Can you work these out from the model? Positions are in its coordinate system, mm. A direction names the side the tool comes from. Coordinates: 2 decimals unless noted, no trailing zeros. Loops run counter-clockwise (first coordinate to the right, second up) from the corner with the lowest first, then second, coordinate; pieces in that order, holes last. Notation, with made-up numbers: M 72.25,-2 L 121.25,-2 A22 cw 121.25,11 Z; hole C 7.5,40 d10. An arc over 180 degrees is marked long. Answer as a JSON object with one key per item and string values. Group by question number.
Item 1: Suppose I cut it at B-B (z = 17.25). Write out the boundary of the cut face in (x, y), then the cut area to 3 significant figures.
Item 2: We'd pull the mould along X, two halves only. Please class faces 4 (the flat face through (-6, 18.562, 15)), 5 (the flat face through (11, -7, 2)), 6 (the cylindrical face through (63.75, 1.4, 4.44)): +X half, -X half, draft (parallel to the pull), parting line (faces both ways), or undercut.
Item 3: Suppose I cut it at C-C (x = -7.5). Write out the boundary of the cut face in (y, z).
Item 4: I'm going to push flat-ended pins straight in: pin 1 Ø8 at (y, z) = (-8, 4.5) entering from -X; pin 2 Ø6.5 at (x, y) = (25, 0) entering from -Z; pin 3 Ø1.2 at (y, z) = (10, 3.5) entering from -X; pin 4 Ø3 at (x, z) = (19, 3.5) entering from -Y. Where does each tip first touch, or does it pass through?
Item 5: If I drill on line 1 (X direction, y = -3.5, z = 14.25); line 2 (Y direction, x = 62.25, z = 13.5); line 3 (Y direction, x = 48, z = 2.5), over which ranges is the centre line in solid material (lowest first)?
Item 6: Suppose I cut it at D-D (x = 62.25). Write out the boundary of the cut face in (y, z).
Item 7: Which directions (+Z, -Z, +X, -X, +Y, -Y) give clear straight access to the entire face, cutting with the end or side of a thin tool? Please do faces 1 (the flat face through (12, 9.062, 7)), 2 (the flat face through (39, 2, 12)), 3 (the flat face through (11, 10, 6)).
Item 8: Suppose I cut it at A-A (x = -29.75). Write out the boundary of the cut face in (y, z).
```python
from build123d import *

# Parameters (mm, degrees)
SKETCH1_W           = 100
SKETCH1_H           = 40
BOSS_EXTRUDE1_DEPTH = 38
CUT_EXTRUDE2_START  = -12
SKETCH2_W           = 39.5
SKETCH2_H           = 34
CUT_EXTRUDE2_DEPTH  = 21
CUT_EXTRUDE4_REACH  = 81.36
SKETCH4_R           = 1.45
SKETCH6_W           = 100
SKETCH6_H           = 19
CUT_EXTRUDE5_DEPTH  = 87.215210375
FILLET1_R           = 0.5
CUT_EXTRUDE12_DEPTH = 9
CUT_EXTRUDE13_REACH = 72.385
SKETCH18_R          = 2.506862912
SKETCH18_R_2        = 2.693115416
SKETCH19_R          = 6.477
SKETCH19_R_2        = 4.572
CUT_EXTRUDE14_DEPTH = 0.79375
SKETCH21_W          = 10
SKETCH21_H          = 15
CUT_EXTRUDE15_DEPTH = 9
SKETCH22_W          = 4
SKETCH22_H          = 2.5
CUT_EXTRUDE16_DEPTH = 90
SKETCH23_W          = 80
SKETCH23_H          = 6
CUT_EXTRUDE17_DEPTH = 9


with BuildPart() as part:
    # Sketch1 → Boss-Extrude1 (new body)
    with BuildSketch(Plane.XY):
        with Locations((16.25, 1.5625)):
            Rectangle(SKETCH1_W, SKETCH1_H)
    extrude(amount=BOSS_EXTRUDE1_DEPTH)

    # Sketch2 → Cut-Extrude2 (cut)
    with BuildSketch(Plane(origin=(0, 0, 0), x_dir=(-1, 0, 0), z_dir=(0, 0, -1)).offset(CUT_EXTRUDE2_START)):
        with Locations((-38.5, 1.5625)):
            Rectangle(SKETCH2_W, SKETCH2_H)
        with Locations((6, 1.5625)):
            Rectangle(SKETCH2_W, SKETCH2_H)
    extrude(amount=-CUT_EXTRUDE2_DEPTH, mode=Mode.SUBTRACT)

    # Sketch4 → Cut-Extrude4 (cut, up to next)
    with BuildSketch(Plane(origin=(0, 0, 0), x_dir=(-1, 0, 0), z_dir=(0, 0, -1)), mode=Mode.PRIVATE) as cut_extrude4_sk1:
        with Locations((-62.25, 16.0625)):
            Circle(SKETCH4_R)
    cut_extrude4_tool1 = extrude(cut_extrude4_sk1.sketch, amount=-CUT_EXTRUDE4_REACH, mode=Mode.PRIVATE) & part.part
    # Sketch4 → Cut-Extrude4 (cut, up to next)
    with BuildSketch(Plane(origin=(0, 0, 0), x_dir=(-1, 0, 0), z_dir=(0, 0, -1)), mode=Mode.PRIVATE) as cut_extrude4_sk2:
        with Locations((-62.25, -12.9375)):
            Circle(SKETCH4_R)
    cut_extrude4_tool2 = extrude(cut_extrude4_sk2.sketch, amount=-CUT_EXTRUDE4_REACH, mode=Mode.PRIVATE) & part.part
    # Sketch4 → Cut-Extrude4 (cut, up to next)
    with BuildSketch(Plane(origin=(0, 0, 0), x_dir=(-1, 0, 0), z_dir=(0, 0, -1)), mode=Mode.PRIVATE) as cut_extrude4_sk3:
        with Locations((29.75, 16.0625)):
            Circle(SKETCH4_R)
    cut_extrude4_tool3 = extrude(cut_extrude4_sk3.sketch, amount=-CUT_EXTRUDE4_REACH, mode=Mode.PRIVATE) & part.part
    # Sketch4 → Cut-Extrude4 (cut, up to next)
    with BuildSketch(Plane(origin=(0, 0, 0), x_dir=(-1, 0, 0), z_dir=(0, 0, -1)), mode=Mode.PRIVATE) as cut_extrude4_sk4:
        with Locations((29.75, -12.9375)):
            Circle(SKETCH4_R)
    cut_extrude4_tool4 = extrude(cut_extrude4_sk4.sketch, amount=-CUT_EXTRUDE4_REACH, mode=Mode.PRIVATE) & part.part
    add(cut_extrude4_tool1.solids().sort_by_distance((62.25, 16.0625, 0))[0], mode=Mode.SUBTRACT)
    add(cut_extrude4_tool2.solids().sort_by_distance((62.25, -12.9375, 0))[0], mode=Mode.SUBTRACT)
    add(cut_extrude4_tool3.solids().sort_by_distance((-29.75, 16.0625, 0))[0], mode=Mode.SUBTRACT)
    add(cut_extrude4_tool4.solids().sort_by_distance((-29.75, -12.9375, 0))[0], mode=Mode.SUBTRACT)

    # Sketch6 → Cut-Extrude5 (cut, through all)
    with BuildSketch(Plane(origin=(0, 21.5625, 0), x_dir=(1, 0, 0), z_dir=(0, 1, 0))):
        with Locations((16.25, -28.5)):
            Rectangle(SKETCH6_W, SKETCH6_H)
    extrude(amount=-CUT_EXTRUDE5_DEPTH, mode=Mode.SUBTRACT)

    # Fillet1
    fillet1_edges = [part.edges().sort_by_distance(p)[0] for p in [
        (-25.75, -15.4375, 15.5),
        (13.75, -15.4375, 15.5),
        (-25.75, 18.5625, 15.5),
        (13.75, 18.5625, 15.5),
        (18.75, -15.4375, 15.5),
        (58.25, -15.4375, 15.5),
        (18.75, 18.5625, 15.5),
        (58.25, 18.5625, 15.5),
    ]]
    fillet(fillet1_edges, radius=FILLET1_R)

    # Sketch17 → Cut-Extrude12 (cut)
    with BuildSketch(Plane(origin=(0, 0, 0), x_dir=(-1, 0, 0), z_dir=(0, 0, -1))):
        with BuildLine():
            Line((-56.25, 9.0625), (23.75, 9.0625))
            ThreePointArc((23.75, 9.0625), (31.25, 1.5625), (23.75, -5.9375))
            Line((23.75, -5.9375), (-56.25, -5.9375))
            ThreePointArc((-56.25, -5.9375), (-63.75, 1.5625), (-56.25, 9.0625))
        make_face()
    extrude(amount=-CUT_EXTRUDE12_DEPTH, mode=Mode.SUBTRACT)

    # Sketch18 → Cut-Extrude13 (cut, up to next)
    with BuildSketch(Plane(origin=(0, 0, 9), x_dir=(-1, 0, 0), z_dir=(0, 0, -1)), mode=Mode.PRIVATE) as cut_extrude13_sk1:
        with Locations((-26.25, 1.5625)):
            Circle(SKETCH18_R)
    cut_extrude13_tool1 = extrude(cut_extrude13_sk1.sketch, amount=-CUT_EXTRUDE13_REACH, mode=Mode.PRIVATE) & part.part
    # Sketch18 → Cut-Extrude13 (cut, up to next)
    with BuildSketch(Plane(origin=(0, 0, 9), x_dir=(-1, 0, 0), z_dir=(0, 0, -1)), mode=Mode.PRIVATE) as cut_extrude13_sk2:
        with Locations((-6.25, 1.5625)):
            Circle(SKETCH18_R_2)
    cut_extrude13_tool2 = extrude(cut_extrude13_sk2.sketch, amount=-CUT_EXTRUDE13_REACH, mode=Mode.PRIVATE) & part.part
    add(cut_extrude13_tool1.solids().sort_by_distance((26.25, 1.5625, 9))[0], mode=Mode.SUBTRACT)
    add(cut_extrude13_tool2.solids().sort_by_distance((6.25, 1.5625, 9))[0], mode=Mode.SUBTRACT)

    # Sketch19 → Cut-Extrude14 (cut)
    # profile 1 of 2: a face of its own
    with BuildSketch(Plane(origin=(0, 0, 9), x_dir=(-1, 0, 0), z_dir=(0, 0, -1))):
        with Locations((-26.25, 1.5625)):
            Circle(SKETCH19_R)
        with Locations((-26.25, 1.5625)):
            Circle(SKETCH19_R_2, mode=Mode.SUBTRACT)
    # profile 2 of 2: a face of its own
    with BuildSketch(Plane(origin=(0, 0, 9), x_dir=(-1, 0, 0), z_dir=(0, 0, -1))):
        with Locations((-6.25, 1.5625)):
            Circle(SKETCH19_R)
        with Locations((-6.25, 1.5625)):
            Circle(SKETCH19_R_2, mode=Mode.SUBTRACT)
    extrude(amount=-CUT_EXTRUDE14_DEPTH, mode=Mode.SUBTRACT)

    # Sketch21 → Cut-Extrude15 (cut)
    with BuildSketch(Plane(origin=(0, 0, 0), x_dir=(-1, 0, 0), z_dir=(0, 0, -1))):
        with Locations((28.75, 1.5625)):
            Rectangle(SKETCH21_W, SKETCH21_H)
    extrude(amount=-CUT_EXTRUDE15_DEPTH, mode=Mode.SUBTRACT)

    # Sketch22 → Cut-Extrude16 (cut)
    with BuildSketch(Plane.ZY.offset(33.75)):
        with Locations((4, 10.3125)):
            Rectangle(SKETCH22_W, SKETCH22_H)
        with Locations((4, -7.1875)):
            Rectangle(SKETCH22_W, SKETCH22_H)
    extrude(amount=-CUT_EXTRUDE16_DEPTH, mode=Mode.SUBTRACT)

    # Sketch23 → Cut-Extrude17 (cut)
    with BuildSketch(Plane(origin=(0, 0, 0), x_dir=(-1, 0, 0), z_dir=(0, 0, -1))):
        with Locations((-16.25, 18.5625)):
            Rectangle(SKETCH23_W, SKETCH23_H)
        with Locations((-16.25, -15.4375)):
            Rectangle(SKETCH23_W, SKETCH23_H)
    extrude(amount=-CUT_EXTRUDE17_DEPTH, mode=Mode.SUBTRACT)


solid = part.part
```
From the geometry:
{
 "1": {"outline": "M -33.75,-18.44 L 66.25,-18.44 L 66.25,21.56 L -33.75,21.56 Z; hole C -29.75,-12.94 d2.9; hole C -29.75,16.06 d2.9; hole M -25.75,-14.94 A0.5 ccw -25.25,-15.44 L 13.25,-15.44 A0.5 ccw 13.75,-14.94 L 13.75,18.06 A0.5 ccw 13.25,18.56 L -25.25,18.56 A0.5 ccw -25.75,18.06 Z; hole M 18.75,-14.94 A0.5 ccw 19.25,-15.44 L 57.75,-15.44 A0.5 ccw 58.25,-14.94 L 58.25,18.06 A0.5 ccw 57.75,18.56 L 19.25,18.56 A0.5 ccw 18.75,18.06 Z; hole C 62.25,-12.94 d2.9; hole C 62.25,16.06 d2.9", "area": "1,290 mm2"},
 "2": {"face 4": "undercut", "face 5": "draft", "face 6": "-X half"},
 "3": {"outline": "M -18.44,9 L -12.44,9 L -12.44,0 L -5.94,0 L -5.94,2 L -8.44,2 L -8.44,6 L -5.94,6 L -5.94,9 L 9.06,9 L 9.06,6 L 11.56,6 L 11.56,2 L 9.06,2 L 9.06,0 L 15.56,0 L 15.56,9 L 21.56,9 L 21.56,19 L 18.56,19 L 18.56,12 L -15.44,12 L -15.44,19 L -18.44,19 Z"},
 "4": {"pin 1": "x = -33.75", "pin 2": "z = 9", "pin 3": "x = 56.25", "pin 4": "y = -12.44"},
 "5": {"line 1": "-33.75 to -25.75, 13.75 to 18.75, 58.25 to 66.25", "line 2": "-18.44 to -14.39, -11.49 to 14.61, 17.51 to 21.56", "line 3": "-12.44 to -8.44, 11.56 to 15.56"},
 "6": {"outline": "M -18.44,0 L -14.39,0 L -14.39,19 L -18.44,19 Z; M -11.49,0 L -2.94,0 L -2.94,9 L 6.06,9 L 6.06,0 L 14.61,0 L 14.61,19 L -11.49,19 Z; M 17.51,0 L 21.56,0 L 21.56,19 L 17.51,19 Z"},
 "7": {"face 1": "-Z, -X", "face 2": "+Z", "face 3": "-X"},
 "8": {"outline": "M -18.44,0 L -14.39,0 L -14.39,19 L -18.44,19 Z; M -11.49,0 L -5.94,0 L -5.94,2 L -8.44,2 L -8.44,6 L -5.94,6 L -5.94,9 L 9.06,9 L 9.06,6 L 11.56,6 L 11.56,2 L 9.06,2 L 9.06,0 L 14.61,0 L 14.61,19 L -11.49,19 Z; M 17.51,0 L 21.56,0 L 21.56,19 L 17.51,19 Z"}
}
